```python
from build123d import *

# Parameters (mm, degrees)
SKIZZE1_W                       = 110
SKIZZE1_H                       = 230
AUFSATZ_LINEAR_AUSTRAGEN1_DEPTH = 4
M3_GEWINDEBOHRUNG1_D            = 2.5
DURCHGANGSLOCH_F_R_M41_D        = 4.3
DURCHGANGSLOCH_F_R_M33_DEPTH    = 4
DURCHGANGSLOCH_F_R_M32_D        = 3.4
SKIZZE10_R                      = 11
SCHNITT_LINEAR_AUSTRAGEN1_DEPTH = 128.538229563
DURCHGANGSLOCH_F_R_M42_D        = 4.5
FASE1_SIZE                      = 3


# Read off the part's stored shape, not the designer's step: Durchgangsloch für M33
with BuildPart() as part:
    # Skizze1 → Aufsatz-Linear austragen1 (new body)
    with BuildSketch(Plane.XY):
        Rectangle(SKIZZE1_W, SKIZZE1_H)
    extrude(amount=AUFSATZ_LINEAR_AUSTRAGEN1_DEPTH)

    # M3 Gewindebohrung1 (through all)
    with Locations(Plane.XY.offset(4)):
        with Locations((-16, 65), (-16, 25), (-16, -15), (-16, -55)):
            Hole(M3_GEWINDEBOHRUNG1_D / 2)

    # Durchgangsloch für M41 (through all)
    with Locations(Plane.XY.offset(4)):
        with Locations((-45, 105), (45, 105), (-45, 45), (-45, -15), (45, 45), (45, -15), (45, -75), (-45, -75)):
            Hole(DURCHGANGSLOCH_F_R_M41_D / 2)

    # Durchgangsloch für M33 outline → Durchgangsloch für M33 (cut)
    with BuildSketch(Plane.XY):
        with BuildLine():
            Line((-8.8, 83.7), (-8.8, 86.3))
            ThreePointArc((-8.8, 86.3), (-10.5, 88), (-12.2, 86.3))
            Line((-12.2, 86.3), (-12.2, 83.7))
            ThreePointArc((-12.2, 83.7), (-10.5, 82), (-8.8, 83.7))
        make_face()
        with BuildLine():
            ThreePointArc((-8.8, -73.7), (-10.5, -72), (-12.2, -73.7))
            Line((-12.2, -73.7), (-12.2, -76.3))
            ThreePointArc((-12.2, -76.3), (-10.5, -78), (-8.8, -76.3))
            Line((-8.8, -76.3), (-8.8, -73.7))
        make_face()
        with BuildLine():
            Line((-19.8, 83.7), (-19.8, 86.3))
            ThreePointArc((-19.8, 86.3), (-21.5, 88), (-23.2, 86.3))
            Line((-23.2, 86.3), (-23.2, 83.7))
            ThreePointArc((-23.2, 83.7), (-21.5, 82), (-19.8, 83.7))
        make_face()
        with BuildLine():
            ThreePointArc((-19.8, -73.7), (-21.5, -72), (-23.2, -73.7))
            Line((-23.2, -73.7), (-23.2, -76.3))
            ThreePointArc((-23.2, -76.3), (-21.5, -78), (-19.8, -76.3))
            Line((-19.8, -76.3), (-19.8, -73.7))
        make_face()
    extrude(amount=DURCHGANGSLOCH_F_R_M33_DEPTH, mode=Mode.SUBTRACT)

    # Durchgangsloch für M32 (through all)
    with Locations(Plane.XY.offset(4)):
        with Locations((21.899494937, -80.100505063), (2.100505063, -80.100505063), (21.899494937, -99.899494937), (2.100505063, -99.899494937)):
            Hole(DURCHGANGSLOCH_F_R_M32_D / 2)

    # Skizze10 → Schnitt-Linear austragen1 (cut, through all)
    with BuildSketch(Plane.XY.offset(4)):
        with Locations((12, -90)):
            Circle(SKIZZE10_R)
    extrude(amount=-SCHNITT_LINEAR_AUSTRAGEN1_DEPTH, mode=Mode.SUBTRACT)

    # Durchgangsloch für M42 (through all)
    with Locations(Plane.XY.offset(4)):
        with Locations((12, 100)):
            Hole(DURCHGANGSLOCH_F_R_M42_D / 2)

    # Fase1
    fase1_edges = [part.edges().sort_by_distance(p)[0] for p in [
        (-55, 115, 2),
        (55, 115, 2),
        (55, -115, 2),
        (-55, -115, 2),
    ]]
    chamfer(fase1_edges, length=FASE1_SIZE)


solid = part.part
```
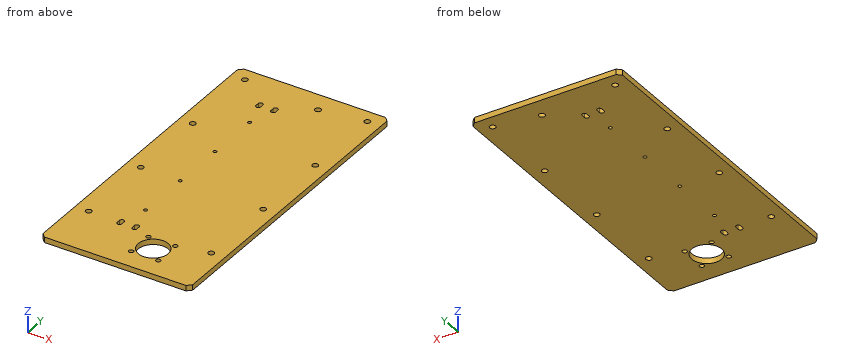
Source: CAD feature listing. Evaluate the final solid. Frame: model axes, mm. Coordinates: 2 decimals unless noted, no trailing zeros. Write each loop counter-clockwise with the first axis right and the second up, starting at its lowest first coordinate (ties: lowest second). Pieces come first, ordered by that corner, then holes. Notation, with made-up numbers: M 45,60 L 54,60 A12 cw 54,79 Z; hole C 64.5,7 d1. An arc over 180 degrees is marked long. Answer as a JSON object with one key per item and string values.
1. Cut plane C-C on z = 3.3. State how many separate pieces and enclosed holes the cut face has, plus the area to 3 significant figures.
Evaluation:
{"separate pieces": "1", "enclosed holes": "22", "area": "24,600 mm^2"}
2. Cut plane A-A on y = 100. Output: boundary loops of the cut face in (x, z).
Evaluation:
{"outline": "M -55,0 L 9.75,0 L 9.75,4 L -55,4 Z; M 14.25,0 L 55,0 L 55,4 L 14.25,4 Z"}
3. Cut plane B-B on x = 12. Output: boundary loops of the cut face in (y, z).
Evaluation:
{"outline": "M -115,0 L -101,0 L -101,4 L -115,4 Z; M -79,0 L 97.75,0 L 97.75,4 L -79,4 Z; M 102.25,0 L 115,0 L 115,4 L 102.25,4 Z"}
4. Ray query, L1, parallel to Y at x = -45, z = 1.9; L2, parallel to Y at x = 11, z = 3.05; L3, parallel to Y at x = 21.5, z = 2.8. Return the intervals inside material, ascending.
Evaluation:
{"L1": "-115 to -77.15, -72.85 to -17.15, -12.85 to 42.85, 47.15 to 102.85, 107.15 to 115", "L2": "-115 to -100.95, -79.05 to 97.98, 102.02 to 115", "L3": "-115 to -101.55, -98.25 to -95.55, -84.45 to -81.75, -78.45 to 115"}
